Solid Edge part; units mm, degrees
sketch "Sketch1" plane through (0, 0, 0) normal (1, 0, 0) x (0, 1, 0)
  line L0 (-17.8191, 46.8648) -> (-17.8191, 6.8648)
  line L1 (-17.8191, 6.8648) -> (-57.8191, 6.8648)
  line L2 (-57.8191, 6.8648) -> (-57.8191, 11.8648)
  line L3 (-57.8191, 11.8648) -> (-22.8191, 11.8648)
  line L4 (-22.8191, 11.8648) -> (-22.8191, 46.8648)
  line L5 (-22.8191, 46.8648) -> (-17.8191, 46.8648)
  dimension "D1" = 57.8191
  dimension "D2" = 22.8191
  dimension "D3" = 17.8191
  dimension "D4" = 17.8191
extrude "Protrusion1" add sketch "Sketch1" against normal blind 100
sketch "Sketch2" plane through (-50, -22.8191, 29.3648) normal (0, -1, 0) x (1, 0, 0)
  circle A0 centre (30, 0) radius 5
  circle A1 centre (-30, 0) radius 5
extrude "Cutout1" cut sketch "Sketch2" against normal through all
mirror "Mirror1" about plane through (-50, -35.1934, 24.2392) normal (0, -0.7071, -0.7071) of "Cutout1"
The listing builds one solid part. Answer for the finished solid, in the listing's coordinates (mm). A direction names the side the tool comes from. Coordinates: 2 decimals unless noted, no trailing zeros. Write each loop counter-clockwise with the first axis right and the second up, starting at its lowest first coordinate (ties: lowest second). Pieces come first, ordered by that corner, then holes. Notation, with made-up numbers: (-1, 60.25) - (28, 60.25) arc R14 ccw to (28, 68.25) - close; hole circle Ø1 at (46, 85.5). An arc over 180 degrees is marked (long way). Return JSON: item names as keys, results as strings. Group by question number.
1. Given pin 1 (10 mm diameter, centred on x = -39.5, y = -32.5, fed in from +Z); pin 2 (13 mm diameter, centred on x = -20, z = 29.36, fed in from -Y); pin 3 (1 mm diameter, centred on y = -22, z = 18, fed in from +X), each flat-ended and moving along its own axis, determine where each tip first touches the part or whether it passes through.
2. Determine the mould class of faces 3 (the cylindrical face through (-75.38, -42.23, 9.4)), 4 (the cylindrical face through (-21.08, -45.2, 9.4)), 5 (the flat face through (-49, -17.819, 27)), 6 (the cylindrical face through (-23.69, -20.35, 32.74)) for opening direction Y: released by +Y, released by -Y, zero draft, split by the parting line, or undercut.
3. A cutting plane is placed at B-B, the plane x = -6.5. Determine the outline of the cut face in (y, z).
4. Which of the six approach directions +Z, -Z, +X, -X, +Y, -Y give full straight-line access (tool end or side, diameter ignored) to faces 1 (the flat face through (-49, -41, 11.865)), 2 (the flat face through (-49, -38, 6.865))?
5. Straight lines are drawn through the part: L1, parallel to Y at x = -20, z = 8; L2, parallel to Z at x = -80, y = -18.85; L3, parallel to Y at x = -38.5, z = 27. For each, find the intervals that lie inside material, in ascending order.
6. A cutting plane is placed at D-D, the plane y = -24. Determine the outline of the cut face in (x, z).
7. A cutting plane is placed at C-C, the plane z = 23. Determine the outline of the cut face in (x, y), plus the area to 3 significant figures.
8. A cutting plane is placed at A-A, the plane x = -20. Determine the outline of the cut face in (y, z), plus the area to 3 significant figures.
Ans:
{
 "1": {"pin 1": "z = 11.86", "pin 2": "y = -22.82", "pin 3": "x = 0"},
 "2": {"face 3": "undercut", "face 4": "undercut", "face 5": "released by +Y", "face 6": "zero draft"},
 "3": {"outline": "(-57.82, 6.86) - (-17.82, 6.86) - (-17.82, 46.86) - (-22.82, 46.86) - (-22.82, 11.86) - (-57.82, 11.86) - close"},
 "4": {"face 1": "+Z, +X, -X, -Y", "face 2": "-Z, +X, -X, +Y, -Y"},
 "5": {"L1": "-57.82 to -45.32, -35.32 to -17.82", "L2": "6.86 to 24.36, 34.36 to 46.86", "L3": "-22.82 to -17.82"},
 "6": {"outline": "(-100, 6.86) - (0, 6.86) - (0, 11.86) - (-100, 11.86) - close"},
 "7": {"outline": "(-100, -22.82) - (0, -22.82) - (0, -17.82) - (-100, -17.82) - close", "area": "500 mm²"},
 "8": {"outline": "(-57.82, 6.86) - (-45.32, 6.86) - (-45.32, 11.86) - (-57.82, 11.86) - close; (-35.32, 6.86) - (-17.82, 6.86) - (-17.82, 24.36) - (-22.82, 24.36) - (-22.82, 11.86) - (-35.32, 11.86) - close; (-22.82, 34.36) - (-17.82, 34.36) - (-17.82, 46.86) - (-22.82, 46.86) - close", "area": "275 mm²"}
}
